from build123d import *

# Parameters (mm, degrees)
BOSS_EXTRUDE1_DEPTH = 20
BOSS_EXTRUDE2_DEPTH = 4
SKETCH3_R           = 2
CUT_EXTRUDE1_DEPTH  = 30.2
SKETCH4_R           = 1.5
CUT_EXTRUDE2_DEPTH  = 2


with BuildPart() as part:
    # Sketch1 → Boss-Extrude1 (new body)
    with BuildSketch(Plane(origin=(0, 0, 0), x_dir=(1, 0, 0), z_dir=(0, 1, 0))):
        Polygon((0, 0), (0, 40.5), (-26, 40.5), (-26, 47.5), (-29.2, 47.5), (-29.2, 40.5), (-33.031373033, 40.5), (-37, 36), (-37, 24), (-36, 23.118082896), (-36, 0), (-29.2, 0), (-29.2, -7), (-26, -7), (-26, 0), align=None)
    extrude(amount=BOSS_EXTRUDE1_DEPTH)

    # Sketch2 → Boss-Extrude2 (add)
    with BuildSketch(Plane.ZY.offset(37)):
        Polygon((-33.464101615, 10), (-31.732050808, 7), (-28.267949192, 7), (-26.535898385, 10), (-28.267949192, 13), (-31.732050808, 13), align=None)
    extrude(amount=BOSS_EXTRUDE2_DEPTH)

    # Sketch3 → Cut-Extrude1 (cut, through all)
    with BuildSketch(Plane.ZY.offset(29.2)):
        with Locations((-45, 5.2)):
            Circle(SKETCH3_R)
        with Locations((-45, 14.8)):
            Circle(SKETCH3_R)
        with Locations((4.5, 14.8)):
            Circle(SKETCH3_R)
        with Locations((4.5, 5.2)):
            Circle(SKETCH3_R)
    extrude(amount=-CUT_EXTRUDE1_DEPTH, mode=Mode.SUBTRACT)

    # Sketch4 → Cut-Extrude2 (cut)
    with BuildSketch(Plane.ZY.offset(41)):
        with Locations((-30, 10)):
            Circle(SKETCH4_R)
    extrude(amount=-CUT_EXTRUDE2_DEPTH, mode=Mode.SUBTRACT)


solid = part.part
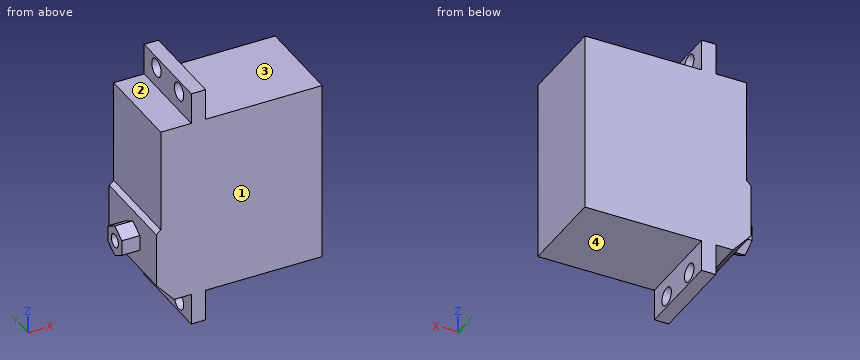
Build history of the part. All positions in model axes, mm. Face numbers are marked on the shaded views. A direction names the side the tool comes from. Coordinates: 2 decimals unless noted, no trailing zeros. Order: outer loops, then holes, each group sorted by start corner. A loop starts at its lowest first (then second) coordinate and runs counter-clockwise, first axis right, second up. Notation, with made-up numbers: (-20.5, 30) - (-1.5, 30) arc R12 ccw to (-1.5, 51) - close; hole circle Ø2 at (89.25, 40). An arc over 180 degrees is marked (long way). Put each result on its own line as item: value.
1. Saw through at A-A (z = -45). Write the cut outline in (x, y).
Answer sheet:
outline: (-29.2, 0) - (-26, 0) - (-26, 3.2) - (-29.2, 3.2) - close; (-29.2, 7.2) - (-26, 7.2) - (-26, 12.8) - (-29.2, 12.8) - close; (-29.2, 16.8) - (-26, 16.8) - (-26, 20) - (-29.2, 20) - close
2. Saw through at B-B (y = 14.8). Write the cut outline in (x, z), and give its area (3 significant figures).
Answer sheet:
outline: (-37, -36) - (-33.03, -40.5) - (-29.2, -40.5) - (-29.2, -43) - (-26, -43) - (-26, -40.5) - (0, -40.5) - (0, 0) - (-26, 0) - (-26, 2.5) - (-29.2, 2.5) - (-29.2, 0) - (-36, 0) - (-36, -23.12) - (-37, -24) - close; (-29.2, -47.5) - (-26, -47.5) - (-26, -47) - (-29.2, -47) - close; (-29.2, 6.5) - (-26, 6.5) - (-26, 7) - (-29.2, 7) - close
area: 1,490 mm^2
3. Tool access for the marked faces 1, 2, 3 and 4: list every direction of +Z, -Z, +X, -X, +Y, -Y with a clear straight run to the whole face (end or side of a thin tool).
Answer sheet:
face 1: +Z, -Z, +X, -X, -Y
face 2: +Z, -X, +Y, -Y
face 3: +Z, +X, +Y, -Y
face 4: -Z, +X, +Y, -Y
4. Drop flat-ended pins along their axis: P1, Ø6.5, axis at y = 5.2, z = 4.5, coming from the -X side; P2, Ø4.5, axis at y = 5.2, z = -45, coming from the +X side; P3, Ø5.5, axis at x = -33, y = 10, coming from the +Z side. Give the stop position or say it passes through.
Answer sheet:
P1: stops at x = -29.2
P2: stops at x = -26
P3: stops at z = 0
5. Probe line 1 along Z through (x, y) = (-26.5, 15.5); line 2 along Y through (x, z) = (-28.25, 4.5); line 3 along Z through (x, y) = (-27, 16.5). List the from-to ranges inside material, lowest first. Write a range as [from, to].
Answer sheet:
line 1: z = [-47.5, -46.87], [-43.13, 2.63], [6.37, 7]
line 2: y = [0, 3.2], [7.2, 12.8], [16.8, 20]
line 3: z = [-47.5, -46.05], [-43.95, 3.45], [5.55, 7]
6. Saw through at C-C (x = -31.5). Write the cut outline in (y, z), and give its area (3 significant figures).
Answer sheet:
outline: (0, -40.5) - (20, -40.5) - (20, 0) - (0, 0) - close
area: 810 mm^2
7. Saw through at D-D (z = -18). Write the cut outline in (x, y), and give its area (3 significant figures).
Answer sheet:
outline: (-36, 0) - (0, 0) - (0, 20) - (-36, 20) - close
area: 720 mm^2
